Part model, mm, in its own coordinate system. Give positions to 0.01 mm unless a question says otherwise; leave off trailing zeros. Order: outer loops, then holes, each group sorted by start corner. A loop starts at its lowest first (then second) coordinate and runs counter-clockwise, first axis right, second up. Notation, with made-up numbers: (-14.5, -19) - (34.5, -19) arc R13 ccw to (34.5, -8) - close; hole circle Ø8 at (52.25, 74). An arc over 180 degrees is marked (long way). Use one line per item in the form item = value. Start each with the question number.
1. Band-saw the part on A-A, the plane z = 14. List the corners of the cut face in (x, y).
2. Band-saw the part on B-B, the plane x = -8.5. List the corners of the cut face in (y, z).
3. Pin check, flat tips, straight feed: P1, Ø1.3, axis at x = 0, y = 5, coming from the -Z side; P2, Ø1.2, axis at x = -6, y = -3.5, coming from the +Z side; P3, Ø7.5, axis at x = 8.5, z = 2.5, coming from the +Y side. Stop position of each tip, or through.
4. Band-saw the part on D-D, the plane y = 3.5. List the corners of the cut face in (x, z).
5. Drill centre lines: line 1 (X direction, y = -3, z = -14.5); line 2 (Y direction, x = 7.5, z = 9); line 3 (Y direction, x = -0.5, z = 13.5). Where is each one in solid material? Low to high.
6. Band-saw the part on C-C, the plane z = -4. List the corners of the cut face in (x, y).
from build123d import *

# Parameters (mm, degrees)
F0_W      = 25.4
F0_H      = 50
F1_DEPTH  = 7.62
F2_W      = 7.112
F2_H      = 2.54
F3_DEPTH  = 1.27
F3_FACE_W = 7.112
F3_FACE_H = 2.54
F4_DEPTH  = 1.27
F6_DEPTH  = 2.54
F7_W      = 7
F7_H      = 2.5
F8_DEPTH  = 40


with BuildPart() as f1:
    # F0 (on Front) → F1 (new body)
    with BuildSketch(Plane.XZ):
        Rectangle(F0_W, F0_H)
    extrude(amount=F1_DEPTH)

    # F2 (on Right) → F3 (join)
    with BuildSketch(Plane.YZ):
        with Locations((3.556, 23.73)):
            Rectangle(F2_W, F2_H)
    extrude(amount=F3_DEPTH)

    # F3_face (on face) → F4 (join)
    with BuildSketch(Plane(origin=(0, 3.556, 23.73), x_dir=(0, 1, 0), z_dir=(-1, 0, 0))):
        Rectangle(F3_FACE_W, F3_FACE_H)
    extrude(amount=F4_DEPTH)

    # F5 (on face) → F6 (join)
    with BuildSketch(Plane(origin=(-1.27, 0, 0), x_dir=(0, -1, 0), z_dir=(-1, 0, 0))):
        Polygon((-7.112, 22.46), (-7.112, 25), (-10.112, 25), (-10.112, -0.4), (-7.112, -0.4), align=None)
    extrude(amount=-F6_DEPTH)

    # F7 (on face) → F8 (cut)
    with BuildSketch(Plane.XY.offset(25)):
        with Locations((-6.956602, -3.36)):
            Rectangle(F7_W, F7_H)
        with Locations((7.587198, -3.36)):
            Rectangle(F7_W, F7_H)
    extrude(amount=-F8_DEPTH, mode=Mode.SUBTRACT)


solid = f1.part
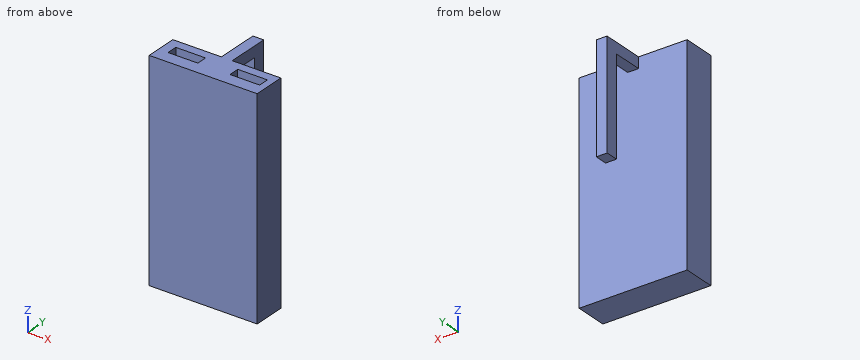
From the geometry:
q1.outline = (-12.7, -7.62) - (12.7, -7.62) - (12.7, 0) - (-12.7, 0) - close; (-1.27, 7.11) - (1.27, 7.11) - (1.27, 10.11) - (-1.27, 10.11) - close; hole (-10.46, -4.61) - (-3.46, -4.61) - (-3.46, -2.11) - (-10.46, -2.11) - close; hole (4.09, -4.61) - (11.09, -4.61) - (11.09, -2.11) - (4.09, -2.11) - close
q2.outline = (-7.62, -25) - (0, -25) - (0, 25) - (-2.11, 25) - (-2.11, -15) - (-4.61, -15) - (-4.61, 25) - (-7.62, 25) - close
q3.P1 = 22.46
q3.P2 = -15
q3.P3 = 0
q4.outline = (-1.27, 22.46) - (1.27, 22.46) - (1.27, 25) - (-1.27, 25) - close
q5.line_1 = -12.7 to -10.46, -3.46 to 4.09, 11.09 to 12.7
q5.line_2 = -7.62 to -4.61, -2.11 to 0
q5.line_3 = -7.62 to 0, 7.11 to 10.11
q6.outline = (-12.7, -7.62) - (12.7, -7.62) - (12.7, 0) - (-12.7, 0) - close; hole (-10.46, -4.61) - (-3.46, -4.61) - (-3.46, -2.11) - (-10.46, -2.11) - close; hole (4.09, -4.61) - (11.09, -4.61) - (11.09, -2.11) - (4.09, -2.11) - close
